Work out the finished part from the listing and answer in its coordinate system (mm). Face numbers are marked on the shaded views. A direction names the side the tool comes from. Round coordinates to 2 decimals unless told otherwise and drop trailing zeros. Loops run counter-clockwise (first coordinate to the right, second up) from the corner with the lowest first, then second, coordinate; pieces in that order, holes last.
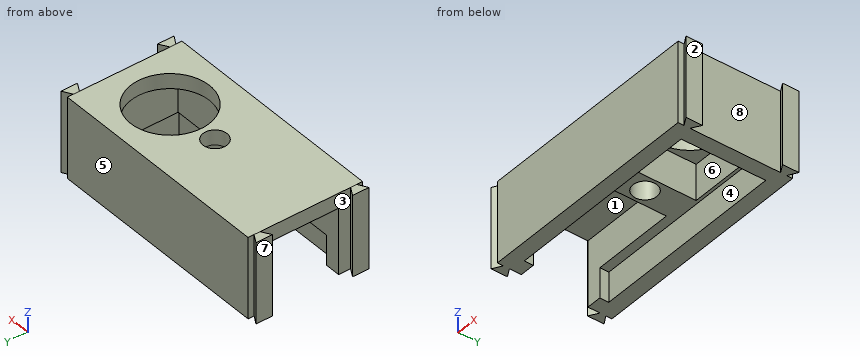
```python
from build123d import *

# Parameters (mm, degrees)
SKETCH2_W           = 38
SKETCH2_H           = 19.1
SKETCH2_R           = 6.55
SKETCH2_R_2         = 2
BOSS_EXTRUDE1_DEPTH = 2.5
SKETCH3_R           = 2
SKETCH3_W           = 13.5
SKETCH3_H           = 13.1
BOSS_EXTRUDE2_DEPTH = 6
BOSS_EXTRUDE3_DEPTH = 5
BOSS_EXTRUDE4_DEPTH = 13.5


with BuildPart() as part:
    # Sketch2 → Boss-Extrude1 (new body)
    with BuildSketch(Plane.XY):
        Rectangle(SKETCH2_W, SKETCH2_H)
        with Locations((9.45, 0)):
            Circle(SKETCH2_R, mode=Mode.SUBTRACT)
        Circle(SKETCH2_R_2, mode=Mode.SUBTRACT)
    extrude(amount=-BOSS_EXTRUDE1_DEPTH)

    # Sketch3 → Boss-Extrude2 (add)
    with BuildSketch(Plane(origin=(0, 0, -2.5), x_dir=(-1, 0, 0), z_dir=(0, 0, -1))):
        Polygon((-19, -9.55), (19, -9.55), (19, -5.55), (2.5, -5.55), (2.5, 5.55), (19, 5.55), (19, 9.55), (-19, 9.55), align=None)
        with Locations(Location((0, 0, 0), (0, 0, 180))):
            Circle(SKETCH3_R, mode=Mode.SUBTRACT)
        with Locations((-9.25, 0)):
            Rectangle(SKETCH3_W, SKETCH3_H, mode=Mode.SUBTRACT)
    extrude(amount=BOSS_EXTRUDE2_DEPTH)

    # Sketch4 → Boss-Extrude3 (add)
    with BuildSketch(Plane(origin=(0, 0, -8.5), x_dir=(-1, 0, 0), z_dir=(0, 0, -1))):
        Polygon((19, 5.55), (16.5, 5.55), (16.5, 7.05), (-16.5, 7.05), (-16.5, -7.05), (16.5, -7.05), (16.5, -5.55), (19, -5.55), (19, -9.55), (-19, -9.55), (-19, 9.55), (19, 9.55), align=None)
    extrude(amount=BOSS_EXTRUDE3_DEPTH)

    # Sketch5 → Boss-Extrude4 (add)
    with BuildSketch(Plane(origin=(0, 0, -13.5), x_dir=(-1, 0, 0), z_dir=(0, 0, -1))):
        Polygon((-19, 8.55), (-20.5, 9.416025404), (-20.5, 6.683974596), (-19, 7.55), align=None)
        Polygon((-19, -7.55), (-19, -8.55), (-20.5, -9.416025404), (-20.5, -6.683974596), align=None)
    boss_extrude4 = extrude(amount=-BOSS_EXTRUDE4_DEPTH)

    # Mirror1: Boss-Extrude4 across plane
    add(boss_extrude4.mirror(Plane(origin=(0, 0, 0), x_dir=(0, 0, 1), z_dir=(1, 0, 0))))


solid = part.part
```
1. Find section A-A (x = 0). Write down the section's boundary in (y, z), then the cut area to 3 significant figures.
Answer key:
outline: (-9.55, -13.5) - (-7.05, -13.5) - (-7.05, -8.5) - (-2, -8.5) - (-2, 0) - (-9.55, 0) - close; (2, -8.5) - (7.05, -8.5) - (7.05, -13.5) - (9.55, -13.5) - (9.55, 0) - (2, 0) - close
area: 153 mm2
2. Find section B-B (z = -1.5). Write down the section's boundary in (x, y).
Answer key:
outline: (-20.5, -9.42) - (-19, -8.55) - (-19, -9.55) - (19, -9.55) - (19, -8.55) - (20.5, -9.42) - (20.5, -6.68) - (19, -7.55) - (19, 7.55) - (20.5, 6.68) - (20.5, 9.42) - (19, 8.55) - (19, 9.55) - (-19, 9.55) - (-19, 8.55) - (-20.5, 9.42) - (-20.5, 6.68) - (-19, 7.55) - (-19, -7.55) - (-20.5, -6.68) - close; hole circle Ø4 at (0, 0); hole circle Ø13.1 at (9.45, 0)
3. Find section D-D (x = -11). Write down the section's boundary in (y, z), then the cut area to 3 significant figures.
Answer key:
outline: (-9.55, -13.5) - (-7.05, -13.5) - (-7.05, -8.5) - (-5.55, -8.5) - (-5.55, -2.5) - (5.55, -2.5) - (5.55, -8.5) - (7.05, -8.5) - (7.05, -13.5) - (9.55, -13.5) - (9.55, 0) - (-9.55, 0) - close
area: 121 mm2
4. Determine the mould class of the marked faces 5, 6, 7 and 8 for opening direction Y: +Y half, -Y half, draft (parallel to the pull), parting line (faces both ways), or undercut.
Answer key:
face 5: +Y half
face 6: undercut
face 7: draft
face 8: undercut
5. Which of the six approach directions +Z, -Z, +X, -X, +Y, -Y give full straight-line access (tool end or side, diameter ignored) to the marked faces 1, 2, 3 and 4?
Answer key:
face 1: -Z, -X
face 2: +Z, -Z, +X, +Y, -Y
face 3: +Z, -Z
face 4: -Z
6. Consider probe 1 along Y at (x, z) = (0, -4.55); probe 2 along Y at (x, z) = (9.45, -0.55); probe 3 along X at (y, z) = (2.25, -5). Determine where each line is inside the solid, lowest interval first.
Answer key:
probe 1: y = -9.55 to -2, 2 to 9.55
probe 2: y = -9.55 to -6.55, 6.55 to 9.55
probe 3: x = -2.5 to 2.5, 16 to 19
7. Given pin 1 (5.5 mm diameter, centred on x = -7.5, y = -0.5, fed in from -Z); pin 2 (1.5 mm diameter, centred on y = 2, z = -2.5, fed in from +X); pin 3 (10 mm diameter, centred on x = 1, y = -6.5, fed in from +Z); pin 4 (6.5 mm diameter, centred on y = -3, z = -5.5, fed in from -X), each flat-ended and moving along its own axis, determine where each tip first touches the part or whether it passes through.
Answer key:
pin 1: stops at z = -2.5
pin 2: stops at x = 19
pin 3: stops at z = 0
pin 4: stops at x = -19
8. Find section C-C (y = -0.75). Write down the section's boundary in (x, z), then the cut area to 3 significant figures.
Answer key:
outline: (-19, -2.5) - (-2.5, -2.5) - (-2.5, -8.5) - (-1.85, -8.5) - (-1.85, 0) - (-19, 0) - close; (1.85, -8.5) - (2.5, -8.5) - (2.5, -2.5) - (2.94, -2.5) - (2.94, 0) - (1.85, 0) - close; (15.96, -2.5) - (16, -2.5) - (16, -8.5) - (16.5, -8.5) - (16.5, -13.5) - (19, -13.5) - (19, 0) - (15.96, 0) - close
area: 91.4 mm2
